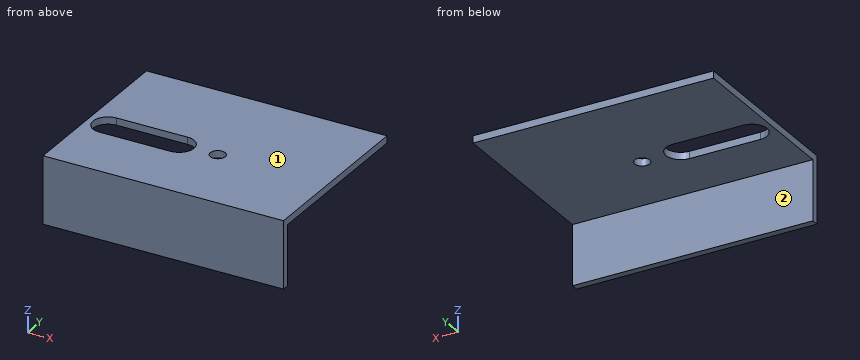
from build123d import *

# Parameters (mm, degrees)
CROQUIS1_W              = 101.6
CROQUIS1_H              = 76.2
SALIENTE_EXTRUIR1_DEPTH = 3
CROQUIS2_W              = 101.6
CROQUIS2_H              = 3
SALIENTE_EXTRUIR2_DEPTH = 25.4
CROQUIS3_R              = 3.175
CORTAR_EXTRUIR1_DEPTH   = 70.561555474


with BuildPart() as part:
    # Croquis1 → Saliente-Extruir1 (new body)
    with BuildSketch(Plane.XY):
        Rectangle(CROQUIS1_W, CROQUIS1_H)
    extrude(amount=SALIENTE_EXTRUIR1_DEPTH)

    # Croquis2 → Saliente-Extruir2 (add)
    with BuildSketch(Plane(origin=(0, 0, 0), x_dir=(-1, 0, 0), z_dir=(0, 0, -1))):
        with Locations((0, -36.6)):
            Rectangle(CROQUIS2_W, CROQUIS2_H)
    extrude(amount=SALIENTE_EXTRUIR2_DEPTH)

    # Croquis3 → Cortar-Extruir1 (cut, through all)
    with BuildSketch(Plane.XY.offset(3)):
        with Locations((4.33, -5.5)):
            Circle(CROQUIS3_R)
        with BuildLine():
            Line((-42.02, 0.85), (-12.02, 0.85))
            ThreePointArc((-12.02, 0.85), (-5.67, -5.5), (-12.02, -11.85))
            Line((-12.02, -11.85), (-42.02, -11.85))
            ThreePointArc((-42.02, -11.85), (-48.37, -5.5), (-42.02, 0.85))
        make_face()
    extrude(amount=-CORTAR_EXTRUIR1_DEPTH, mode=Mode.SUBTRACT)


solid = part.part
Can you work these out from the model? Positions are in its coordinate system, mm. Face numbers are marked on the shaded views. A direction names the side the tool comes from. Round coordinates to 2 decimals unless told otherwise and drop trailing zeros. Write each loop counter-clockwise with the first axis right and the second up, starting at its lowest first coordinate (ties: lowest second). Pieces come first, ordered by that corner, then holes. Notation, with made-up numbers: (66.25, 39) -> (94.25, 39) arc R28 cw to (94.25, 58) -> close; hole circle Ø11 at (7, 25.25). An arc over 180 degrees is marked (long way). Use one line per item in the form item = value. Start each with the question number.
Q1. Imagine slicing it at B-B (y = -5.5). Please give me the cut outline in (x, z) (3 decimals).
Q2. Which directions (+Z, -Z, +X, -X, +Y, -Y) give clear straight access to the entire face, cutting with the end or side of a thin tool? Please do the marked faces 1 and 2.
Q3. Imagine slicing it at D-D (y = -18). Please give me the cut outline in (x, z), then the cut area to 3 significant figures.
Q4. I'm going to push flat-ended pins straight in: P1, Ø12, axis at x = -8, y = -3.5, coming from the -Z side; P2, Ø7.5, axis at x = -3, z = -12, coming from the +Y side; P3, Ø3, axis at x = -9, y = -3, coming from the -Z side. Where does each tip first touch, or does it pass through?
Q5. Imagine slicing it at A-A (x = 4.33). Please give me the cut outline in (y, z) (3 decimals).
Q6. Imagine slicing it at C-C (x = -20). Please give me the cut outline in (y, z), then the cut area to 3 significant figures.
Q7. If I drill on probe 1 along Y at (x, z) = (4.33, 1.4) (3 decimals); probe 2 along Z at (x, y) = (-20, 27.5); probe 3 along Y at (x, z) = (-18.5, -1), over which ranges is the centre line in solid material (lowest first)? Write a range as [from, to].
Worked out:
q1.outline = (-50.8, 0) -> (-48.37, 0) -> (-48.37, 3) -> (-50.8, 3) -> close; (-5.67, 0) -> (1.155, 0) -> (1.155, 3) -> (-5.67, 3) -> close; (7.505, 0) -> (50.8, 0) -> (50.8, 3) -> (7.505, 3) -> close
q2.face_1 = +Z, +X, -X, +Y, -Y
q2.face_2 = -Z, +X, -X, +Y
q3.outline = (-50.8, 0) -> (50.8, 0) -> (50.8, 3) -> (-50.8, 3) -> close
q3.area = 305 mm^2
q4.P1 = 0
q4.P2 = -35.1
q4.P3 = through
q5.outline = (-38.1, -25.4) -> (-35.1, -25.4) -> (-35.1, 0) -> (-8.675, 0) -> (-8.675, 3) -> (-38.1, 3) -> close; (-2.325, 0) -> (38.1, 0) -> (38.1, 3) -> (-2.325, 3) -> close
q6.outline = (-38.1, -25.4) -> (-35.1, -25.4) -> (-35.1, 0) -> (-11.85, 0) -> (-11.85, 3) -> (-38.1, 3) -> close; (0.85, 0) -> (38.1, 0) -> (38.1, 3) -> (0.85, 3) -> close
q6.area = 267 mm^2
q7.probe_1 = [-38.1, -8.675], [-2.325, 38.1]
q7.probe_2 = [0, 3]
q7.probe_3 = [-38.1, -35.1]
